Can you work these out from the model? Positions are in its coordinate system, mm. Coordinates: 2 decimals unless noted, no trailing zeros. Loops run counter-clockwise (first coordinate to the right, second up) from the corner with the lowest first, then second, coordinate; pieces in that order, holes last. Notation, with made-up numbers: M -37,86.25 L -1,86.25 A9 ccw -1,91.25 Z; hole C -34.75,-26 d7. An arc over 180 degrees is marked long. Return JSON: item names as keys, results as strings. Group by question number.
Autodesk Inventor part; units mm, degrees
ref_plane "YZ Plane" through (0, 0, 0) normal (1, 0, 0) x (0, 1, 0)
ref_plane "XZ Plane" through (0, 0, 0) normal (0, 1, 0) x (-1, 0, 0)
ref_plane "XY Plane" through (0, 0, 0) normal (0, 0, 1) x (1, 0, 0)
sketch "Sketch1" plane through (0, 0, 0) normal (0, 1, 0) x (-1, 0, 0)
  line L0 (152.4, 152.4) -> (-152.4, 152.4)
  line L1 (-152.4, 152.4) -> (-152.4, -152.4)
  line L2 (-152.4, -152.4) -> (152.4, -152.4)
  line L3 (152.4, -152.4) -> (152.4, 152.4)
  line L4 (152.4, 152.4) -> (-152.4, -152.4) construction
  line L5 (-152.4, 152.4) -> (152.4, -152.4) construction
  point P0 (0, 0)
  dimension "d0" = 304.8
  dimension "d1" = 304.8
extrude "Plate1" add sketch "Sketch1" along normal blind 3.048
sketch "Sketch2" plane through (0, 3.048, 0) normal (0, 1, 0) x (1, 0, 0)
  line L0 (-152.4, -152.4) -> (152.4, -152.4)
  line L1 (-133.35, -139.7) -> (-41.91, -139.7)
  line L2 (-41.91, -139.7) -> (-41.91, -165.1)
  line L3 (-41.91, -165.1) -> (-133.35, -165.1)
  line L4 (-133.35, -165.1) -> (-133.35, -139.7)
  line L5 (-133.35, -139.7) -> (-41.91, -165.1) construction
  line L6 (-41.91, -139.7) -> (-133.35, -165.1) construction
  line L7 (41.91, -139.7) -> (133.35, -139.7)
  line L8 (133.35, -139.7) -> (133.35, -165.1)
  line L9 (133.35, -165.1) -> (41.91, -165.1)
  line L10 (41.91, -165.1) -> (41.91, -139.7)
  line L11 (41.91, -139.7) -> (133.35, -165.1) construction
  line L12 (133.35, -139.7) -> (41.91, -165.1) construction
  line L13 (-152.4, -152.4) -> (-152.4, 152.4)
  line L14 (152.4, 152.4) -> (152.4, -152.4)
  point P0 (0, 0)
  point P1 (-87.63, -152.4)
  point P2 (87.63, -152.4)
  dimension "d7" = 91.44
  dimension "d8" = 25.4
  dimension "d9" = 91.44
  dimension "d10" = 25.4
  dimension "d11" = 19.05
  dimension "d12" = 19.05
extrude "Cut1" cut sketch "Sketch2" against normal blind 3.048
sketch "Sketch3" plane through (0, 3.048, 0) normal (0, 1, 0) x (1, 0, 0)
  line L0 (-110.49, -119.888) -> (-64.77, -119.888) construction
  line L1 (-110.49, -116.078) -> (-64.77, -116.078)
  line L2 (-64.77, -123.698) -> (-110.49, -123.698)
  arc A0 (-110.49, -116.078) -> (-110.49, -123.698) centre (-110.49, -119.888) ccw
  arc A1 (-64.77, -123.698) -> (-64.77, -116.078) centre (-64.77, -119.888) ccw
  line L3 (-152.4, -152.4) -> (-152.4, 152.4)
  line L4 (-133.35, -139.7) -> (-41.91, -139.7)
  line L5 (-41.91, -152.4) -> (41.91, -152.4) construction
  line L6 (0, -152.4) -> (0, 0) construction
  line L7 (110.49, -119.888) -> (64.77, -119.888) construction
  line L8 (110.49, -116.078) -> (64.77, -116.078)
  line L9 (64.77, -123.698) -> (110.49, -123.698)
  arc A2 (110.49, -123.698) -> (110.49, -116.078) centre (110.49, -119.888) ccw
  arc A3 (64.77, -116.078) -> (64.77, -123.698) centre (64.77, -119.888) ccw
  point P0 (-87.63, -119.888)
  point P1 (87.63, -119.888)
  dimension "d13" = 41.91
  dimension "d14" = 45.72
  dimension "d15" = 3.81
  dimension "d16" = 19.812
extrude "Cut2" cut sketch "Sketch3" against normal blind 3.048
equation "\"d5\" = Thickness"
equation "\"d17\" = Thickness"
equation "\"d2\" = Thickness"
equation "\"BendRadius\" = Thickness"
equation "\"BendReliefWidth\" = Thickness"
equation "\"BendReliefDepth\" = 0.5 * Thickness"
equation "\"CornerReliefSize\" = 4 * Thickness"
equation "\"MinimumRemnant\" = 2 * Thickness"
equation "\"TransitionRadius\" = BendRadius"
equation "\"JacobiRadiusSize\" = BendRadius"
equation "\"GapSize\" = Thickness"
properties part number "FreePanel"
1) Suppose I cut it at B-B, the plane x = 85. List the corners of the cut face in (y, z) for me.
2) For pin 1 (1.5 mm diameter, centred on x = 70, y = 2, fed in from +Z), with a flat end and sliding along its axis, tell me the tip position at first contact or that it passes through.
3) Suppose I cut it at C-C, the plane x = 121.5. List the corners of the cut face in (y, z) for me, then the cut area to 3 significant figures.
4) If I drill on line 1 (Z direction, x = 76.5, y = 1.7); line 2 (Z direction, x = -52.5, y = 2.45); line 3 (Z direction, x = 63.5, y = 0.75), over which ranges is the centre line in solid material (lowest first)? Write a range as from..to.
5) Suppose I cut it at A-A, the plane y = 0.65. List the corners of the cut face in (x, z) for me.
Returned:
{
 "1": {"outline": "M 0,-152.4 L 3.05,-152.4 L 3.05,116.08 L 0,116.08 Z; M 0,123.7 L 3.05,123.7 L 3.05,139.7 L 0,139.7 Z"},
 "2": {"pin 1": "stops at z = 139.7"},
 "3": {"outline": "M 0,-152.4 L 3.05,-152.4 L 3.05,139.7 L 0,139.7 Z", "area": "890 mm²"},
 "4": {"line 1": "z = -152.4..116.08, 123.7..139.7", "line 2": "z = -152.4..139.7", "line 3": "z = -152.4..116.3, 123.48..139.7"},
 "5": {"outline": "M -152.4,-152.4 L 152.4,-152.4 L 152.4,152.4 L 133.35,152.4 L 133.35,139.7 L 41.91,139.7 L 41.91,152.4 L -41.91,152.4 L -41.91,139.7 L -133.35,139.7 L -133.35,152.4 L -152.4,152.4 Z; hole M -110.49,116.08 L -64.77,116.08 A3.81 ccw -64.77,123.7 L -110.49,123.7 A3.81 ccw Z; hole M 64.77,116.08 L 110.49,116.08 A3.81 ccw 110.49,123.7 L 64.77,123.7 A3.81 ccw Z"}
}
